Job drawing, mm, ordinate dimensions from the low corner. One solid piece. Coordinates: 2 decimals unless noted, no trailing zeros. Write item = value, one per line. Start each with the question number.
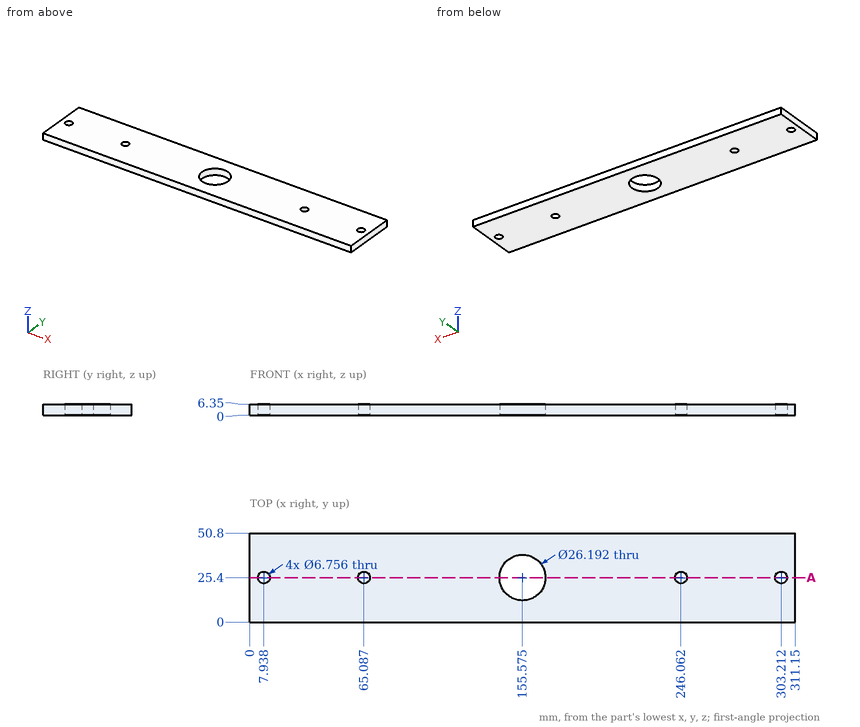
Item 1: Wall check: line 1 along Y through (x, z) = (167.5, 5.75) (1 decimal); line 2 along X through (y, z) = (29, 5.25). Give the ranges that are in metal, low to high. Write a range as [from, to].
Item 2: Flat gauge pin, fed straight in: pin 1 (6 mm diameter, centred on x = 246.06, y = 25.4, fed in from +Z). Where does the tip first touch, or does it go through?
Item 3: Cut at A-A, the plane y = 25.4. Count the separate pieces of the cut face and the enclosed holes in it, and give its area (3 significant figures).
Filled sheet:
q1.line_1 = [0, 20], [30.8, 50.8]
q1.line_2 = [0, 142.98], [168.17, 311.15]
q2.pin_1 = through
q3.separate_pieces = 6
q3.enclosed_holes = 0
q3.area = 1,640 mm2
